```python
from build123d import *

# Parameters (mm, degrees)
SKETCH1_W               = 50.45
SKETCH1_H               = 53.04
BOSS_EXTRUDE1_DEPTH     = 8
CUT_EXTRUDE1_DEPTH      = 6
CUT_EXTRUDE2_DEPTH      = 6
CUT_EXTRUDE3_DEPTH      = 6
CUT_EXTRUDE4_DEPTH      = 6
CUT_EXTRUDE5_DEPTH      = 21
CUT_EXTRUDE5_DEPTH_BACK = 19
SKETCH6_W               = 64.45
SKETCH6_H               = 67.04


with BuildPart() as part:
    # Sketch1 → Boss-Extrude1 (new body)
    with BuildSketch(Plane(origin=(0, 0, 0), x_dir=(1, 0, 0), z_dir=(0, 1, 0))):
        Polygon((50.45, 60.04), (57.45, 60.04), (57.45, 53.04), (57.45, 0), (57.45, -7), (50.45, -7), (0, -7), (-7, -7), (-7, 53.04), (-7, 60.04), (0, 60.04), align=None)
        with Locations((25.225, 26.52)):
            Rectangle(SKETCH1_W, SKETCH1_H, mode=Mode.SUBTRACT)
    extrude(amount=BOSS_EXTRUDE1_DEPTH)

    # Sketch2 → Cut-Extrude1 (cut)
    with BuildSketch(Plane.XY.offset(7)):
        Polygon((-7, 7), (72.572595869, 7), (72.572595869, 1), (-15.083079444, 1), (-15.083079444, 7), align=None)
    extrude(amount=-CUT_EXTRUDE1_DEPTH, mode=Mode.SUBTRACT)

    # Sketch3 → Cut-Extrude2 (cut)
    with BuildSketch(Plane.ZY.offset(7)):
        Polygon((1, 7), (-62.487898414, 7), (-62.487898414, 1), (1, 1), (11.114700275, 1), (11.114700275, 7), align=None)
    extrude(amount=-CUT_EXTRUDE2_DEPTH, mode=Mode.SUBTRACT)

    # Sketch4 → Cut-Extrude3 (cut)
    with BuildSketch(Plane(origin=(0, 0, -60.04), x_dir=(-1, 0, 0), z_dir=(0, 0, -1))):
        Polygon((1, 7), (-63.689958153, 7), (-63.689958153, 1), (1, 1), (11.838030302, 1), (11.838030302, 7), align=None)
    extrude(amount=-CUT_EXTRUDE3_DEPTH, mode=Mode.SUBTRACT)

    # Sketch5 → Cut-Extrude4 (cut)
    with BuildSketch(Plane(origin=(57.45, 0, 0), x_dir=(0, 0, -1), z_dir=(1, 0, 0))):
        Polygon((-1, 7), (54.04, 7), (62.072343262, 7), (62.072343262, 1), (-1, 1), (-8.754047033, 1), (-8.754047033, 7), align=None)
    extrude(amount=-CUT_EXTRUDE4_DEPTH, mode=Mode.SUBTRACT)

    # Sketch6 → Cut-Extrude5 (cut, two sides: drawn at the far end of the back side and taken through both)
    with BuildSketch(Plane(origin=(0, 8, 0), x_dir=(1, 0, 0), z_dir=(0, 1, 0)).offset(-CUT_EXTRUDE5_DEPTH_BACK)):
        with Locations((25.225, 26.52)):
            Rectangle(SKETCH6_W, SKETCH6_H)
        Polygon((-4.150556557, 26.52), (-4.150556557, 57.19), (54.6, 57.19), (54.6, -4.15), (-4.150556557, -4.15), align=None, mode=Mode.SUBTRACT)
    extrude(amount=CUT_EXTRUDE5_DEPTH + CUT_EXTRUDE5_DEPTH_BACK, mode=Mode.SUBTRACT)


solid = part.part
```
Input: part model. Units: mm. Frame: model coordinates. A direction names the side the tool comes from. Coordinates: 2 decimals unless noted, no trailing zeros. Loops run counter-clockwise (first coordinate to the right, second up) from the corner with the lowest first, then second, coordinate; pieces in that order, holes last. Notation, with made-up numbers: M -8.5,74.5 L 17.5,74.5 A13 cw 17.5,94.5 Z; hole C 3,40.25 d7. An arc over 180 degrees is marked long. One line per item, written item: value.
(1) Reachability of faces 1 (the flat face through (50.45, 4, -26)), 2 (the flat face through (26, 4, 1)), 3 (the flat face through (-1, 4, -27)), 4 (the flat face through (-3, 7, -24)) from +Z, -Z, +X, -X, +Y, -Y: full face, straight path, thin tool, end or side. Return the list, or none.
Filled in:
face 1: +Y, -Y
face 2: +Z, +X, -X
face 3: +Z, -Z, -X
face 4: none
(2) Section B-B (x = 36). Output: boundary loops of the cut face in (y, z).
Filled in:
outline: M 0,-57.19 L 1,-57.19 L 1,-54.04 L 7,-54.04 L 7,-57.19 L 8,-57.19 L 8,-53.04 L 0,-53.04 Z; M 0,0 L 8,0 L 8,4.15 L 7,4.15 L 7,1 L 1,1 L 1,4.15 L 0,4.15 Z
(3) Section A-A (y = 4). Output: boundary loops of the cut face in (x, z), and give its area (3 significant figures).
Filled in:
outline: M -1,-54.04 L 51.45,-54.04 L 51.45,1 L -1,1 Z; hole M 0,-53.04 L 50.45,-53.04 L 50.45,0 L 0,0 Z
area: 211 mm^2
(4) Section C-C (z = -25.5). Output: boundary loops of the cut face in (x, y).
Filled in:
outline: M -4.15,0 L 0,0 L 0,8 L -4.15,8 L -4.15,7 L -1,7 L -1,1 L -4.15,1 Z; M 50.45,0 L 54.6,0 L 54.6,1 L 51.45,1 L 51.45,7 L 54.6,7 L 54.6,8 L 50.45,8 Z
(5) Line query: line 1 along X through (y, z) = (6.25, -30); line 2 along Z through (x, y) = (24, 1.5); line 3 along Z through (x, y) = (20, 7.5). Output: solid intervals per line, ascending. Write a range as from..to.
Filled in:
line 1: -1..0, 50.45..51.45
line 2: -54.04..-53.04, 0..1
line 3: -57.19..-53.04, 0..4.15
(6) Pull-direction query (Z, two-part tool) for faces 5 (the flat face through (26, 4, -54.04)), 6 (the flat face through (0, 4, -26)), 7 (the flat face through (51.45, 4, -27)), 8 (the flat face through (25, 4, 0)); classes: +Z half, -Z half, draft (parallel to the pull), parting line (faces both ways), or undercut.
Filled in:
face 5: -Z half
face 6: undercut
face 7: draft
face 8: undercut
(7) Pin query (flat end, axial travel): pin 1 (3 mm diameter, centred on x = 28.5, y = 3.5, fed in from +Z); pin 2 (2.5 mm diameter, centred on y = 3, z = -13.5, fed in from +X); pin 3 (8 mm diameter, centred on x = 46.5, z = -50, fed in from -Y); pin 4 (1.8 mm diameter, centred on y = 3.5, z = -37, fed in from -X). Return the tip coordinate at first contact, or that it passes through.
Filled in:
pin 1: z = 1
pin 2: x = 51.45
pin 3: y = 0
pin 4: x = -1
